```python
from build123d import *

# Parameters (mm, degrees)
SKETCH1_R           = 11
SKETCH1_R_2         = 2.38125
BOSS_EXTRUDE1_DEPTH = 2
SKETCH2_R           = 10.19
SKETCH2_R_2         = 1.1375
BOSS_EXTRUDE2_DEPTH = 1.5
SKETCH3_R           = 10.19
SKETCH3_R_2         = 2.5
BOSS_EXTRUDE3_DEPTH = 1.5
SKETCH5_R           = 11
SKETCH5_R_2         = 2.5
BOSS_EXTRUDE4_DEPTH = 2
SKETCH6_R           = 6.4
SKETCH6_R_2         = 2.5
BOSS_EXTRUDE5_DEPTH = 2
SKETCH7_R           = 11
SKETCH7_R_2         = 2.5
BOSS_EXTRUDE6_DEPTH = 2.4
SKETCH8_R           = 0.5
CUT_EXTRUDE1_DEPTH  = 20.286264542
CHAMFER1_SIZE       = 0.508


with BuildPart() as part:
    # Sketch1 → Boss-Extrude1 (new body)
    with BuildSketch(Plane(origin=(0, 0, 0), x_dir=(1, 0, 0), z_dir=(0, 1, 0))):
        with Locations(Location((0, 0, 0), (0, 0, 270))):
            Circle(SKETCH1_R)
        with Locations(Location((0, 0, 0), (0, 0, 270))):
            Circle(SKETCH1_R_2, mode=Mode.SUBTRACT)
    extrude(amount=BOSS_EXTRUDE1_DEPTH)

    # Sketch2 → Boss-Extrude2 (add)
    with BuildSketch(Plane(origin=(0, 2, 0), x_dir=(1, 0, 0), z_dir=(0, 1, 0))):
        with Locations(Location((0, 0, 0), (0, 0, 270))):
            Circle(SKETCH2_R)
        with Locations(Location((0, 0, 0), (0, 0, 270))):
            Circle(SKETCH2_R_2, mode=Mode.SUBTRACT)
    extrude(amount=BOSS_EXTRUDE2_DEPTH)

    # Sketch3 → Boss-Extrude3 (add)
    with BuildSketch(Plane(origin=(0, 3.5, 0), x_dir=(1, 0, 0), z_dir=(0, 1, 0))):
        with Locations(Location((0, 0, 0), (0, 0, 270))):
            Circle(SKETCH3_R)
        with Locations(Location((0, 0, 0), (0, 0, 270))):
            Circle(SKETCH3_R_2, mode=Mode.SUBTRACT)
    extrude(amount=BOSS_EXTRUDE3_DEPTH)

    # Sketch5 → Boss-Extrude4 (add)
    with BuildSketch(Plane(origin=(0, 5, 0), x_dir=(1, 0, 0), z_dir=(0, 1, 0))):
        with Locations(Location((0, 0, 0), (0, 0, 270))):
            Circle(SKETCH5_R)
        with Locations(Location((0, 0, 0), (0, 0, 270))):
            Circle(SKETCH5_R_2, mode=Mode.SUBTRACT)
    extrude(amount=BOSS_EXTRUDE4_DEPTH)

    # Sketch6 → Boss-Extrude5 (add)
    with BuildSketch(Plane(origin=(0, 7, 0), x_dir=(1, 0, 0), z_dir=(0, 1, 0))):
        with Locations(Location((0, 0, 0), (0, 0, 270))):
            Circle(SKETCH6_R)
        with Locations(Location((0, 0, 0), (0, 0, 270))):
            Circle(SKETCH6_R_2, mode=Mode.SUBTRACT)
    extrude(amount=BOSS_EXTRUDE5_DEPTH)

    # Sketch7 → Boss-Extrude6 (add)
    with BuildSketch(Plane(origin=(0, 9, 0), x_dir=(1, 0, 0), z_dir=(0, 1, 0))):
        with Locations(Location((0, 0, 0), (0, 0, 270))):
            Circle(SKETCH7_R)
        with Locations(Location((0, 0, 0), (0, 0, 270))):
            Circle(SKETCH7_R_2, mode=Mode.SUBTRACT)
    extrude(amount=BOSS_EXTRUDE6_DEPTH)

    # Sketch8 → Cut-Extrude1 (cut, through all)
    with BuildSketch(Plane.XY):
        with Locations(Location((0, 8, 0), (0, 0, 90))):
            Circle(SKETCH8_R)
        with Locations(Location((0, 4, 0), (0, 0, 89.999999996))):
            Circle(SKETCH8_R)
    extrude(amount=-CUT_EXTRUDE1_DEPTH, mode=Mode.SUBTRACT)

    # Chamfer1
    chamfer1_edges = [part.edges().sort_by_distance(p)[0] for p in [
        (0, 7, -11),
        (0, 11.4, -11),
        (0, 9, -11),
        (0, 11.4, -2.5),
        (0, 2, -11),
    ]]
    chamfer(chamfer1_edges, length=CHAMFER1_SIZE)


solid = part.part
```
Could you check a few things on this model? Use its own coordinates, in mm. A direction names the side the tool comes from. Round coordinates to 2 decimals unless told otherwise and drop trailing zeros. Order: outer loops, then holes, each group sorted by start corner. A loop starts at its lowest first (then second) coordinate and runs counter-clockwise, first axis right, second up. Notation, with made-up numbers: (28, 16) -> (57, 16) arc R35 ccw to (57, 49) -> close; hole circle Ø1 at (37, 69). An arc over 180 degrees is marked (long way). One line per question, with ' | ' between items.
Q1. If I drill on line 1 (Y direction, x = 2.5, z = 10); line 2 (Y direction, x = -2, z = -9); line 3 (Z direction, x = -2, y = 6.75), over which ranges is the centre line in solid material (lowest first)? Write a range as from..to.
Computed values:
line 1: 0..2, 5..7, 9..11.4 | line 2: 0..7, 9..11.4 | line 3: -10.55..-1.5, 1.5..10.55
Q2. If we section it at A-A on z = -6.75: Give the number of separate pieces and of enclosed holes in the cut face, plus the area to 3 significant figures.
Computed values:
separate pieces: 2 | enclosed holes: 1 | area: 155 mm²
Q3. If we section it at B-B on y = 1: Write out the boundary of the cut face in (x, z), plus the area to 3 significant figures.
Computed values:
outline: circle Ø22 at (0, 0); hole circle Ø4.76 at (0, 0) | area: 362 mm²
Q4. If we section it at D-D on y = 2.75: Write out the boundary of the cut face in (x, z) (1 decimal), plus the area to 3 significant figures.
Computed values:
outline: circle Ø20.4 at (0, 0); hole circle Ø2.3 at (0, 0) | area: 322 mm²
Q5. I'm going to push flat-ended pins straight in: pin 1 (1.5 mm diameter, centred on x = -6, y = 6, fed in from +Z); pin 2 (2.5 mm diameter, centred on x = 0, z = 0, fed in from +Y); pin 3 (1.5 mm diameter, centred on y = 2.5, z = 1.5, fed in from -X). Where does each tip first touch, or does it pass through?
Computed values:
pin 1: z = 9.67 | pin 2: y = 3.5 | pin 3: x = -10.64
Q6. If we section it at C-C on y = 8: Write out the boundary of the cut face in (x, z).
Computed values:
outline: (-0.5, -6.38) -> (-0.5, -2.45) arc R2.5 cw (long way) to (0.5, -2.45) -> (0.5, -6.38) arc R6.4 ccw (long way) to start
Q7. Which directions (+Z, -Z, +X, -X, +Y, -Y) give clear straight access to the entire face, cutting with the end or side of a thin tool? Please do faces 1 (the face through (5, 7, 5)), 2 (the face through (-0.15, 4.477, -6.266)), 3 (the face through (0.751, 7.144, 2.385)), 4 (the face through (-1.45, 0.99, -1.89)).
Computed values:
face 1: none | face 2: -Z | face 3: +Y | face 4: -Y
Q8. We'd pull the mould along X, two halves only. Please class faces 5 (the face through (-10, 5, 3)), 6 (the face through (-0.15, 8.477, -4.397)), 7 (the face through (1.922, 7.986, 6.104)): released by +X, released by -X, zero draft, split by the parting line, or undercut.
Computed values:
face 5: zero draft | face 6: undercut | face 7: split by the parting line
